Autodesk Inventor part; units mm, degrees
ref_plane "YZ Plane" through (0, 0, 0) normal (1, 0, 0) x (0, 1, 0)
ref_plane "XZ Plane" through (0, 0, 0) normal (0, 1, 0) x (-1, 0, 0)
ref_plane "XY Plane" through (0, 0, 0) normal (0, 0, 1) x (1, 0, 0)
sketch "스케치1" plane through (0, 0, 0) normal (0, 0, 1) x (1, 0, 0)
  line L0 (0, 0) -> (60, 0)
  line L1 (60, 0) -> (60, 70)
  line L2 (60, 70) -> (0, 70)
  line L3 (0, 70) -> (0, 0)
  dimension "d0" = 60
  dimension "d1" = 70
extrude "돌출1" add sketch "스케치1" along normal blind 8
sketch "스케치2" plane through (0, 0, 8) normal (0, 0, 1) x (1, 0, 0)
  line L0 (0, 0) -> (60, 0)
  line L1 (60, 0) -> (60, 70)
  line L2 (60, 70) -> (0, 70)
  line L3 (0, 70) -> (0, 0)
  line L4 (60, 0) -> (60, 70)
  line L5 (0, 70) -> (60, 70)
  line L6 (60, 70) -> (60, 20)
  line L7 (60, 20) -> (0, 20)
  line L8 (0, 20) -> (0, 70)
extrude "돌출2" cut sketch "스케치2" against normal blind 4 contours L3 L2 L1 L7
sketch "스케치3" plane through (0, 0, 4) normal (0, 0, 1) x (1, 0, 0)
  line L0 (60, 70) -> (60, 20)
  line L1 (0, 70) -> (60, 70)
  line L2 (0, 20) -> (0, 70)
  line L3 (60, 20) -> (0, 20)
  line L4 (60, 70) -> (0, 70)
  circle A0 centre (11, 62) radius 1.6
  circle A1 centre (49, 62) radius 1.6
  circle A2 centre (11, 33) radius 1.6
  circle A3 centre (49, 33) radius 1.6
  point P0 (0, 0)
  dimension "d8" = 3.2
  dimension "d9" = 3.2
  dimension "d14" = 3.2
  dimension "d15" = 3.2
  dimension "d16" = 11
  dimension "d17" = 8
  dimension "d18" = 8
  dimension "d19" = 11
  dimension "d20" = 29
  dimension "d21" = 11
  dimension "d22" = 11
  dimension "d23" = 29
extrude "돌출3" cut sketch "스케치3" against normal blind 4 contours A0 | A1 | A2 | A3
sketch "스케치4" plane through (0, 0, 0) normal (0, -1, 0) x (1, 0, 0)
  line L0 (0, 0) -> (60, 0)
  line L1 (60, 0) -> (60, 8)
  line L2 (0, 8) -> (60, 8)
  line L3 (0, 0) -> (0, 8)
extrude "돌출4" cut sketch "스케치4" against normal blind 5
sketch "스케치5" plane through (0, 5, 0) normal (0, -1, 0) x (1, 0, 0)
  circle A0 centre (15, 4) radius 1.5
  circle A1 centre (45, 4) radius 1.5
  line L0 (60, 0) -> (0, 0)
  line L1 (0, 8) -> (60, 8)
  line L2 (0, 0) -> (0, 8)
  line L3 (60, 8) -> (60, 0)
  dimension "d24" = 3
  dimension "d25" = 3
  dimension "d26" = 4
  dimension "d27" = 4
  dimension "d28" = 15
  dimension "d29" = 15
extrude "돌출5" cut sketch "스케치5" against normal blind 8 contours A0 | A1
sketch "스케치6" plane through (0, 0, 8) normal (0, 0, 1) x (1, 0, 0)
  line L0 (16.5, 13) -> (13.5, 13)
  line L1 (16.5, 5) -> (13.5, 5)
  line L2 (46.5, 5) -> (43.5, 5)
  line L3 (46.5, 13) -> (43.5, 13)
  line L4 (46.5, 5) -> (43.5, 5)
  arc A0 (15.6614, 5) -> (14.3386, 5) centre (15, 4.25) ccw
  arc A1 (45.6614, 5) -> (44.3386, 5) centre (45, 4.25) ccw
  point P0 (0, 0)
  dimension "d32" = 2
  dimension "d33" = 2
  dimension "d34" = 0.75
  dimension "d35" = 0.75
extrude "돌출6" cut sketch "스케치6" against normal blind 8
properties part number "앞뒷면PSD받침대" material "ABS 플라스틱"
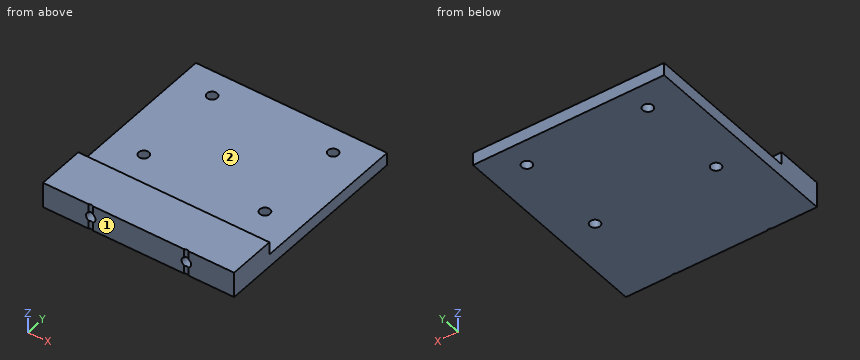
Geometry: final body of the model. Coordinates: model frame, mm. Face numbers are marked on the shaded views. A direction names the side the tool comes from. Round coordinates to 2 decimals unless told otherwise and drop trailing zeros. Order: outer loops, then holes, each group sorted by start corner. A loop starts at its lowest first (then second) coordinate and runs counter-clockwise, first axis right, second up. Notation, with made-up numbers: M -27,14.25 L -4,14.25 A34 cw -4,53.25 Z; hole C 64.5,20 d9. An arc over 180 degrees is marked long. One line per item, written item: value.
(1) Pin query (flat end, axial travel): P1, Ø15, axis at x = 39, y = 49, coming from the +Z side; P2, Ø4.5, axis at x = 16.5, z = 6.5, coming from the +Y side. Return the tip coordinate at first contact, or that it passes through.
Result sheet:
P1: z = 4
P2: y = 20
(2) Cut plane B-B (x = 49). Return the cut outline in (y, z).
Result sheet:
outline: M 5,0 L 31.4,0 L 31.4,4 L 20,4 L 20,8 L 5,8 Z; M 34.6,0 L 60.4,0 L 60.4,4 L 34.6,4 Z; M 63.6,0 L 70,0 L 70,4 L 63.6,4 Z
(3) Line query: probe 1 along Y at (x, z) = (49, 2.3); probe 2 along X at (y, z) = (10.5, 4); probe 3 along Z at (x, y) = (27, 24). Output: solid intervals per line, ascending. Write a range as [from, to].
Result sheet:
probe 1: [5, 31.4], [34.6, 60.4], [63.6, 70]
probe 2: [0, 13.5], [16.5, 43.5], [46.5, 60]
probe 3: [0, 4]
(4) Reachability of the marked faces 1 and 2 from +Z, -Z, +X, -X, +Y, -Y: full face, straight path, thin tool, end or side. Return the list, or none.
Result sheet:
face 1: +Z, -Z, +X, -X, -Y
face 2: +Z, +X, -X, +Y
(5) Cut plane D-D (z = 7). Return the cut outline in (x, y).
Result sheet:
outline: M 0,5 L 14.34,5 A1 cw 15.66,5 L 44.34,5 A1 cw 45.66,5 L 60,5 L 60,20 L 0,20 Z
(6) Cut plane A-A (y = 33). Return the cut outline in (x, z).
Result sheet:
outline: M 0,0 L 9.4,0 L 9.4,4 L 0,4 Z; M 12.6,0 L 47.4,0 L 47.4,4 L 12.6,4 Z; M 50.6,0 L 60,0 L 60,4 L 50.6,4 Z
(7) Cut plane C-C (y = 10.5). Return the cut outline in (x, z), and give its area (3 significant figures).
Result sheet:
outline: M 0,0 L 60,0 L 60,8 L 0,8 Z; hole C 15,4 d3; hole C 45,4 d3
area: 466 mm2
